The listing builds one solid part. Answer for the finished solid, in the listing's coordinates (mm). A direction names the side the tool comes from. Round coordinates to 2 decimals unless told otherwise and drop trailing zeros. Write each loop counter-clockwise with the first axis right and the second up, starting at its lowest first coordinate (ties: lowest second). Pieces come first, ordered by that corner, then holes.
Item 1: Each of these flat-tipped pins is pushed along its axis until it touches: pin 1 (8 mm diameter, centred on x = 0, y = 10, fed in from -Z); pin 2 (3 mm diameter, centred on x = 239, z = 3, fed in from -Y); pin 3 (5 mm diameter, centred on x = 56.5, z = 5, fed in from -Y); pin 4 (3 mm diameter, centred on x = 213.5, z = 6, fed in from +Y). Where does it stop, or does it pass through?
Item 2: Find section B-B on z = 5. Give the vertices of the cut face in (x, y), then the cut area to 3 significant figures.
Item 3: Find section A-A on y = 51.5. Give the vertices of the cut face in (x, z), then the cut area to 3 significant figures.
Item 4: A tool of negligible diameter and unlimited length cuts with its end or side. For faces 1 (the face through (57, 75, 5)), 2 (the face through (252.971, 215, 5)), 3 (the face through (233.921, 89, 5)), from which of +Z, -Z, +X, -X, +Y, -Y can it reach the whole face along a straight path? Write none if from no direction.
Item 5: Find section C-C on x = 82.5. Give the vertices of the cut face in (y, z).
Item 6: Find the intervals of material crossed by probe 1 along X at (y, z) = (98.5, 9.25); probe 2 along X at (y, z) = (29.5, 2); probe 3 along Y at (x, z) = (139, 7.75), in increasing order.
Item 7: Find section D-D on x = 156.5. Give the vertices of the cut face in (y, z).
Autodesk Inventor part; units mm, degrees
ref_plane "YZ Plane" through (0, 0, 0) normal (1, 0, 0) x (0, 1, 0)
ref_plane "XZ Plane" through (0, 0, 0) normal (0, 1, 0) x (-1, 0, 0)
ref_plane "XY Plane" through (0, 0, 0) normal (0, 0, 1) x (1, 0, 0)
sketch "Sketch1" plane through (0, 0, 0) normal (0, 0, 1) x (1, 0, 0)
  line L0 (0, 0) -> (505.9426, 0)
  line L1 (505.9426, 0) -> (505.9426, 98.87)
  line L2 (505.9426, 98.87) -> (0, 98.87)
  line L3 (0, 98.87) -> (0, 0)
  line L4 (0, 98.87) -> (252.9713, 244.923)
  line L5 (252.9713, 244.923) -> (505.9426, 98.87)
  point P0 (252.9713, 98.87)
  dimension "d0" = 505.9426
  dimension "d1" = 98.87
  dimension "d2" = 30
extrude "Extrusion1" add sketch "Sketch1" along normal blind 10
sketch "Sketch2" plane through (0, 0, 10) normal (0, 0, 1) x (1, 0, 0)
  line L0 (0, 98.87) -> (0, 0)
  line L1 (252.9713, 244.923) -> (0, 98.87)
  line L2 (505.9426, 98.87) -> (252.9713, 244.923)
  line L3 (505.9426, 0) -> (505.9426, 98.87)
  line L4 (-10, 0) -> (-10, 104.6435)
  line L5 (-10, 104.6435) -> (252.9713, 256.4701)
  line L6 (252.9713, 256.4701) -> (515.9426, 104.6435)
  line L7 (515.9426, 104.6435) -> (515.9426, 0)
  line L8 (-10, 0) -> (0, 0)
  line L9 (0, 0) -> (505.9426, 0)
  line L10 (505.9426, 0) -> (515.9426, 0)
  dimension "d5" = 10
extrude "Extrusion2" add sketch "Sketch2" against normal blind 10 contours L0 L8 L4 L5 L6 L7 L10 L3 L2 L1
sketch "Sketch3" plane through (0, 0, 10) normal (0, 0, 1) x (1, 0, 0)
  line L0 (252.9713, 256.4701) -> (515.9426, 104.6435)
  line L1 (515.9426, 104.6435) -> (515.9426, 0)
  line L2 (252.9713, 256.4701) -> (515.9426, 256.4701)
  line L3 (515.9426, 256.4701) -> (515.9426, 0)
  line L4 (515.9426, 0) -> (252.9713, 0)
  line L5 (252.9713, 0) -> (252.9713, 256.4701)
  point P0 (0, 0)
extrude "Extrusion3" cut sketch "Sketch3" against normal through all
sketch "Sketch4" plane through (0, 0, 10) normal (0, 0, 1) x (1, 0, 0)
  line L0 (252.9713, 0) -> (252.9713, 256.4701) construction
  line L1 (252.9713, 256.4701) -> (-10, 104.6435) construction
  line L2 (-10, 104.6435) -> (-10, 0) construction
  line L3 (-10, 0) -> (252.9713, 0) construction
  line L4 (0, 98.87) -> (242.9713, 239.1495) construction
  line L5 (242.9713, 239.1495) -> (242.9713, 10) construction
  line L6 (242.9713, 10) -> (0, 10) construction
  line L7 (0, 10) -> (0, 98.87) construction
  circle A0 centre (0, 10) radius 2.5
  circle A1 centre (0, 98.87) radius 2.5
  circle A2 centre (242.9713, 239.1495) radius 2.5
  circle A3 centre (242.9713, 10) radius 2.5
  point P0 (0, 0)
  dimension "d10" = 10
  dimension "d11" = 5
  dimension "d12" = 5
  dimension "d13" = 5
  dimension "d14" = 5
extrude "Extrusion4" cut sketch "Sketch4" against normal through all
sketch "Sketch5" plane through (0, 0, 10) normal (0, 0, 1) x (1, 0, 0)
  line L0 (272.0213, 175) -> (233.9213, 175)
  line L1 (233.9213, 175) -> (233.9213, 0)
  line L2 (233.9213, 0) -> (272.0213, 0)
  line L3 (272.0213, 0) -> (272.0213, 175)
  line L4 (-10, 0) -> (252.9713, 0)
  line L5 (38.1, 0) -> (76.2, 0)
  line L6 (76.2, 0) -> (76.2, 75)
  line L7 (76.2, 75) -> (38.1, 75)
  line L8 (38.1, 75) -> (38.1, 0)
  line L9 (-10, 0) -> (-10, 104.6435)
  point P0 (0, 0)
  point P1 (252.9713, 175)
  dimension "d17" = 38.1
  dimension "d18" = 38.1
  dimension "d19" = 48.1
  dimension "d20" = 75
  dimension "d23" = 175
extrude "Extrusion5" cut sketch "Sketch5" against normal through all
properties part number "BA10" material "ABS Plastic"
Check values:
1. pin 1: stops at z = 0
1. pin 2: stops at y = 175
1. pin 3: stops at y = 75
1. pin 4: stops at y = 234.55
2. outline: (-10, 0) - (38.1, 0) - (38.1, 75) - (76.2, 75) - (76.2, 0) - (233.92, 0) - (233.92, 175) - (252.97, 175) - (252.97, 256.47) - (-10, 104.64) - close; hole circle Ø5 at (0, 10); hole circle Ø5 at (0, 98.87); hole circle Ø5 at (242.97, 239.15)
2. area: 41,200 mm2
3. outline: (-10, 0) - (38.1, 0) - (38.1, 10) - (-10, 10) - close; (76.2, 0) - (233.92, 0) - (233.92, 10) - (76.2, 10) - close
3. area: 2,060 mm2
4. face 1: +Z, -Z, -Y
4. face 2: +Z, -Z, +X, +Y, -Y
4. face 3: +Z, -Z, +X, -Y
5. outline: (0, 0) - (158.05, 0) - (158.05, 10) - (0, 10) - close
6. probe 1: x = -10 to -2.47, 2.47 to 233.92
6. probe 2: x = -10 to 38.1, 76.2 to 233.92
6. probe 3: y = 0 to 190.67
7. outline: (0, 0) - (200.77, 0) - (200.77, 10) - (0, 10) - close
